Can you work these out from the model? Positions are in its coordinate system, mm. Give positions to 0.01 mm unless a question says otherwise; leave off trailing zeros. Order: outer loops, then holes, each group sorted by start corner. A loop starts at its lowest first (then second) coordinate and runs counter-clockwise, first axis right, second up. Notation, with made-up numbers: (64, -35.5) - (76, -35.5) arc R26 cw to (76, 1.5) - close; hole circle Ø1 at (-22.5, 71.25). An arc over 180 degrees is marked (long way). Use one line per item in the form item = value. Start each with the question number.
1) For pin 1 (6 mm diameter, centred on x = 0, y = -36.825, fed in from +Z); pin 2 (6.5 mm diameter, centred on x = 0, y = 36.825, fed in from +Z), each with a flat end and sliding along its axis, tell me the tip position at first contact or that it passes through.
2) Suppose I cut it at A-A, the plane x = 0. Write out the boundary of the cut face in (y, z) (1 decimal), and give its area (3 significant figures).
3) Please list where these lines run through material, in increasing order: probe 1 along Y at (x, z) = (0, 0.25) (3 decimals); probe 2 along Y at (x, z) = (0, 2.5) (3 decimals); probe 3 along X at (y, z) = (-37.5, 0.55) (3 decimals).
4) Suppose I cut it at B-B, the plane y = 0. Write out the boundary of the cut face in (x, z) (3 decimals).
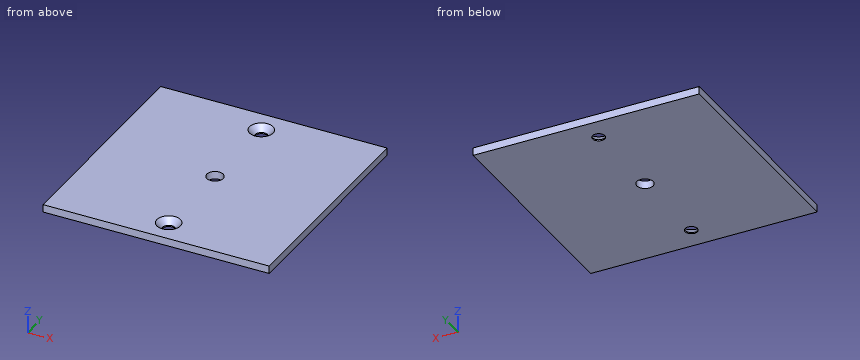
```python
from build123d import *

# Parameters (mm, degrees)
SKETCH1_W                                       = 93.649999898
SKETCH1_H                                       = 93.649999898
BOSS_EXTRUDE1_DEPTH                             = 3.175
F_1_4_CLEARANCE_HOLE1_D                         = 6.7564
F_1_4_CLEARANCE_HOLE1_DEPTH                     = 4.826
F_1_4_CLEARANCE_HOLE1_TIP                       = 2.029827343
CSK_FOR_10_FLAT_HEAD_MACHINE_SCREW1_D           = 5.1054
CSK_FOR_10_FLAT_HEAD_MACHINE_SCREW1_DEPTH       = 4.826
CSK_FOR_10_FLAT_HEAD_MACHINE_SCREW1_CSINK_D     = 9.779
CSK_FOR_10_FLAT_HEAD_MACHINE_SCREW1_CSINK_ANGLE = 82
CSK_FOR_10_FLAT_HEAD_MACHINE_SCREW1_TIP         = 1.533816902


with BuildPart() as part:
    # Sketch1 → Boss-Extrude1 (new body)
    with BuildSketch(Plane.XY):
        Rectangle(SKETCH1_W, SKETCH1_H)
    extrude(amount=BOSS_EXTRUDE1_DEPTH)

    # 1/4 Clearance Hole1
    with Locations(Plane.XY.offset(3.175)):
        with Locations((0, 0)):
            Hole(F_1_4_CLEARANCE_HOLE1_D / 2, depth=F_1_4_CLEARANCE_HOLE1_DEPTH)
            with Locations((0, 0, -(F_1_4_CLEARANCE_HOLE1_DEPTH + F_1_4_CLEARANCE_HOLE1_TIP / 2))):  # 118° drill point
                Cone(0, F_1_4_CLEARANCE_HOLE1_D / 2, F_1_4_CLEARANCE_HOLE1_TIP, mode=Mode.SUBTRACT)

    # CSK for #10 Flat Head Machine Screw1
    with Locations(Plane.XY.offset(3.175)):
        with Locations((0, 36.824999949), (0, -36.824999949)):
            CounterSinkHole(CSK_FOR_10_FLAT_HEAD_MACHINE_SCREW1_D / 2, CSK_FOR_10_FLAT_HEAD_MACHINE_SCREW1_CSINK_D / 2, depth=CSK_FOR_10_FLAT_HEAD_MACHINE_SCREW1_DEPTH, counter_sink_angle=CSK_FOR_10_FLAT_HEAD_MACHINE_SCREW1_CSINK_ANGLE)
            with Locations((0, 0, -(CSK_FOR_10_FLAT_HEAD_MACHINE_SCREW1_DEPTH + CSK_FOR_10_FLAT_HEAD_MACHINE_SCREW1_TIP / 2))):  # 118° drill point
                Cone(0, CSK_FOR_10_FLAT_HEAD_MACHINE_SCREW1_D / 2, CSK_FOR_10_FLAT_HEAD_MACHINE_SCREW1_TIP, mode=Mode.SUBTRACT)


solid = part.part
```
Result sheet:
q1.pin_1 = 1
q1.pin_2 = 1.29
q2.outline = (-46.8, 0) - (-39.4, 0) - (-39.4, 0.5) - (-41.7, 3.2) - (-46.8, 3.2) - close; (-34.3, 0) - (-3.4, 0) - (-3.4, 3.2) - (-31.9, 3.2) - (-34.3, 0.5) - close; (3.4, 0) - (34.3, 0) - (34.3, 0.5) - (31.9, 3.2) - (3.4, 3.2) - close; (39.4, 0) - (46.8, 0) - (46.8, 3.2) - (41.7, 3.2) - (39.4, 0.5) - close
q2.area = 231 mm²
q3.probe_1 = -46.825 to -39.378, -34.272 to -3.378, 3.378 to 34.272, 39.378 to 46.825
q3.probe_2 = -46.825 to -41.128, -32.522 to -3.378, 3.378 to 32.522, 41.128 to 46.825
q3.probe_3 = -46.825 to -2.519, 2.519 to 46.825
q4.outline = (-46.825, 0) - (-3.378, 0) - (-3.378, 3.175) - (-46.825, 3.175) - close; (3.378, 0) - (46.825, 0) - (46.825, 3.175) - (3.378, 3.175) - close
